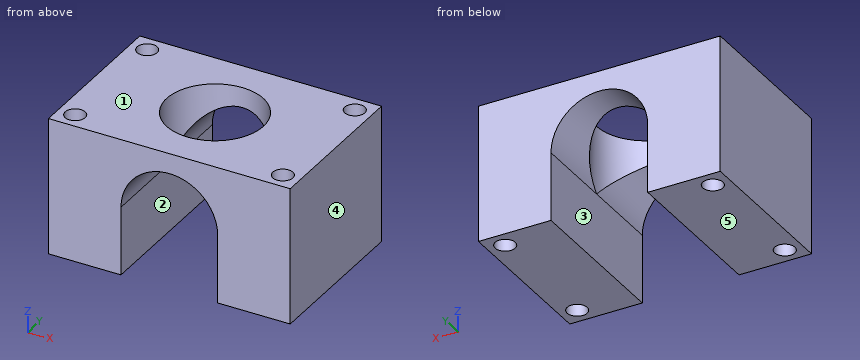
```python
from build123d import *

# Parameters (mm, degrees)
SKETCH1_W           = 60
SKETCH1_H           = 40
BOSS_EXTRUDE1_DEPTH = 34
CUT_EXTRUDE1_DEPTH  = 40
SKETCH3_R           = 12
CUT_EXTRUDE2_DEPTH  = 40
SKETCH4_R           = 2.5
CUT_EXTRUDE3_DEPTH  = 40


with BuildPart() as part:
    # Sketch1 → Boss-Extrude1 (new body)
    with BuildSketch(Plane.XY):
        with Locations((30, 20)):
            Rectangle(SKETCH1_W, SKETCH1_H)
    extrude(amount=BOSS_EXTRUDE1_DEPTH)

    # Sketch2 → Cut-Extrude1 (cut)
    with BuildSketch(Plane.XZ):
        with BuildLine():
            ThreePointArc((42, 17), (30, 29), (18, 17))
            Line((18, 17), (18, 0))
            Line((18, 0), (42, 0))
            Line((42, 0), (42, 17))
        make_face()
    extrude(amount=-CUT_EXTRUDE1_DEPTH, mode=Mode.SUBTRACT)

    # Sketch3 → Cut-Extrude2 (cut)
    with BuildSketch(Plane.XY.offset(34)):
        with Locations((30, 20)):
            Circle(SKETCH3_R)
    extrude(amount=-CUT_EXTRUDE2_DEPTH, mode=Mode.SUBTRACT)

    # Sketch4 → Cut-Extrude3 (cut)
    with BuildSketch(Plane.XY.offset(34)):
        with Locations((55.757359313, 4.242640687)):
            Circle(SKETCH4_R)
        with Locations((4.242640687, 4.242640687)):
            Circle(SKETCH4_R)
        with Locations((55.757359313, 35.757359313)):
            Circle(SKETCH4_R)
        with Locations((4.242640687, 35.757359313)):
            Circle(SKETCH4_R)
    extrude(amount=-CUT_EXTRUDE3_DEPTH, mode=Mode.SUBTRACT)


solid = part.part
```
Model file for the job. Use its own axes, mm. Face numbers are marked on the shaded views. A direction names the side the tool comes from. Give positions to 0.01 mm unless a question says otherwise; leave off trailing zeros. Loops run counter-clockwise (first coordinate to the right, second up) from the corner with the lowest first, then second, coordinate; pieces in that order, holes last. Notation, with made-up numbers: (44, 34) - (97, 34) arc R22 ccw to (97, 66) - close; hole circle Ø1 at (-24.5, 38). An arc over 180 degrees is marked (long way). One line per item, written item: value. Start each with the question number.
1. Pin check, flat tips, straight feed: pin 1 (4.5 mm diameter, centred on x = 55.76, y = 4.24, fed in from +Z); pin 2 (10 mm diameter, centred on x = 36, y = 10, fed in from -Z). Stop position of each tip, or through.
2. Slice it at C-C (y = 11). List the corners of the cut face in (x, z).
3. Probe L1, parallel to X at y = 21, z = 12.5; L2, parallel to Y at x = 55.5, z = 17; L3, parallel to X at y = 4, z = 16. List the from-to ranges inside material, lowest first. Write a range as from..to.
4. Pull direction X, two halves, no side cores. Call the marked faces 3, 4 and 5: pulls with the +X half, pulls with the -X half, needs draft (parallel to the pull), parting line crosses it, or undercut.
5. Which spindle directions (+Z, -Z, +X, -X, +Y, -Y) get a long thin tool onto all of the face, cutting with end or side? Do the marked faces 1 and 2. Say none if no direction does.
6. Slice it at B-B (x = 30). List the corners of the cut face in (y, z), plus the area to 3 significant figures.
7. Slice it at D-D (z = 24.5). List the corners of the cut face in (x, y), plus the area to 3 significant figures.
8. Slice it at A-A (z = 7). List the corners of the cut face in (x, y), plus the area to 3 significant figures.
Solution:
1. pin 1: passes through
1. pin 2: stops at z = 21.8
2. outline: (0, 0) - (18, 0) - (18, 17) arc R12 cw to (22.06, 26) - (22.06, 34) - (0, 34) - close; (37.94, 26) arc R12 cw to (42, 17) - (42, 0) - (60, 0) - (60, 34) - (37.94, 34) - close
3. L1: x = 0..18, 42..60
3. L2: y = 0..1.76, 6.73..33.27, 38.24..40
3. L3: x = 0..1.75, 6.73..18, 42..53.27, 58.25..60
4. face 3: undercut
4. face 4: pulls with the +X half
4. face 5: needs draft
5. face 1: +Z, +X, -X, +Y, -Y
5. face 2: -Z, +Y, -Y
6. outline: (0, 29) - (8, 29) - (8, 34) - (0, 34) - close; (32, 29) - (40, 29) - (40, 34) - (32, 34) - close
6. area: 80.0 mm^2
7. outline: (0, 0) - (20.63, 0) - (20.63, 12.5) arc R12 cw to (20.63, 27.5) - (20.63, 40) - (0, 40) - close; (39.37, 0) - (60, 0) - (60, 40) - (39.37, 40) - (39.37, 27.5) arc R12 cw to (39.37, 12.5) - close; hole circle Ø5 at (4.24, 4.24); hole circle Ø5 at (4.24, 35.76); hole circle Ø5 at (55.76, 4.24); hole circle Ø5 at (55.76, 35.76)
7. area: 1,520 mm^2
8. outline: (0, 0) - (18, 0) - (18, 40) - (0, 40) - close; (42, 0) - (60, 0) - (60, 40) - (42, 40) - close; hole circle Ø5 at (4.24, 4.24); hole circle Ø5 at (4.24, 35.76); hole circle Ø5 at (55.76, 4.24); hole circle Ø5 at (55.76, 35.76)
8. area: 1,360 mm^2
